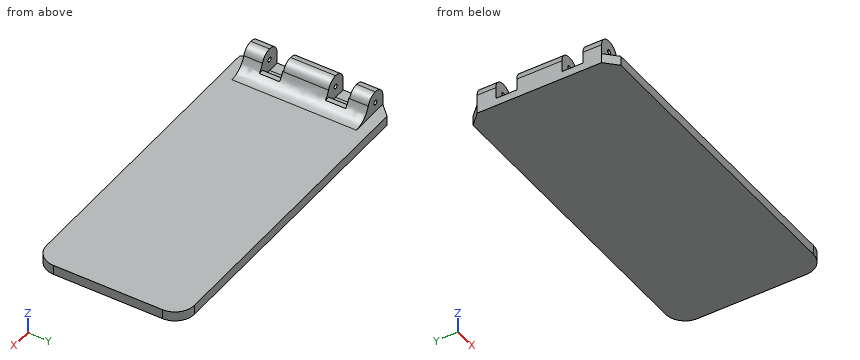
from build123d import *

# Parameters (mm, degrees)
BOSS_EXTRUDE1_DEPTH     = 38
FILLET1_R               = 5
CUT_EXTRUDE2_DEPTH      = 2.7
CUT_EXTRUDE2_DEPTH_BACK = 2.7
SKETCH4_R               = 3
CUT_EXTRUDE3_DEPTH      = 2.7
CUT_EXTRUDE3_DEPTH_BACK = 2.7
SKETCH5_R               = 3
SKETCH6_W               = 15.806991546
SKETCH6_H               = 7.262468959
CUT_EXTRUDE4_DEPTH      = 3
SKETCH7_W               = 28.198471628
SKETCH7_H               = 7.72700603
CUT_EXTRUDE5_DEPTH      = 3
CHAMFER1_SIZE           = 3
FILLET2_R               = 5
SKETCH8_W               = 6.878152115
SKETCH8_H               = 5.2
SKETCH8_W_2             = 6.400502662
CUT_EXTRUDE6_DEPTH      = 2


with BuildPart() as part:
    # Sketch1 → Boss-Extrude1 (new body)
    with BuildSketch(Plane(origin=(0, 0, 0), x_dir=(1, 0, 0), z_dir=(0, 1, 0))):
        with BuildLine():
            Line((85, 0), (3, 0))
            Line((3, 0), (3, -2))
            ThreePointArc((3, -2), (3.866025404, -2.127718677), (4.658312395, -2.5))
            Line((4.658312395, -2.5), (85, -2.5))
            Line((85, -2.5), (85, 0))
        make_face()
        with BuildLine():
            Line((3, -2), (3, 0))
            Line((3, 0), (0, 0))
            Line((0, 0), (0, -2.5))
            Line((0, -2.5), (1.341687605, -2.5))
            ThreePointArc((1.341687605, -2.5), (2.133974596, -2.127718677), (3, -2))
        make_face()
        with BuildLine():
            ThreePointArc((0, -5), (0.356617963, -3.581362835), (1.341687605, -2.5))
            Line((1.341687605, -2.5), (0, -2.5))
            Line((0, -2.5), (0, -5))
        make_face()
        with BuildLine():
            Line((3, -4.4), (3, -2.5))
            Line((3, -2.5), (0, -5))
            ThreePointArc((0, -5), (0.878679656, -7.121320344), (3, -8))
            Line((3, -8), (3, -5.6))
            ThreePointArc((3, -5.6), (2.4, -5), (3, -4.4))
        make_face()
        with BuildLine():
            Line((4.658312395, -2.5), (3, -2.5))
            Line((3, -2.5), (3, -4.4))
            ThreePointArc((3, -4.4), (3.424264069, -4.575735931), (3.6, -5))
            ThreePointArc((3.6, -5), (3.424264069, -5.424264069), (3, -5.6))
            Line((3, -5.6), (3, -8))
            ThreePointArc((3, -8), (5.121320344, -7.121320344), (6, -5))
            ThreePointArc((6, -5), (5.643382037, -3.581362835), (4.658312395, -2.5))
        make_face()
        with BuildLine():
            Line((0, -5), (3, -2.5))
            Line((3, -2.5), (1.341687605, -2.5))
            ThreePointArc((1.341687605, -2.5), (0.356617963, -3.581362835), (0, -5))
        make_face()
        with BuildLine():
            Line((3, -2.5), (3, -2))
            ThreePointArc((3, -2), (2.133974596, -2.127718677), (1.341687605, -2.5))
            Line((1.341687605, -2.5), (3, -2.5))
        make_face()
        with BuildLine():
            ThreePointArc((4.658312395, -2.5), (3.866025404, -2.127718677), (3, -2))
            Line((3, -2), (3, -2.5))
            Line((3, -2.5), (4.658312395, -2.5))
        make_face()
    extrude(amount=BOSS_EXTRUDE1_DEPTH)

    # Fillet1
    fillet1_edges = [part.edges().sort_by_distance(p)[0] for p in [
        (4.658312395, 19, 2.5),
    ]]
    fillet(fillet1_edges, radius=FILLET1_R)

    # Sketch4 → Cut-Extrude2 (cut, two sides: drawn at the far end of the back side and taken through both)
    with BuildSketch(Plane(origin=(0, 27.5, 0), x_dir=(1, 0, 0), z_dir=(0, 1, 0)).offset(-CUT_EXTRUDE2_DEPTH_BACK)):
        with Locations((3, -5)):
            Circle(SKETCH4_R)
        with BuildLine():
            ThreePointArc((0, -5), (0.878679656, -2.878679656), (3, -2))
            Line((3, -2), (0, -2))
            Line((0, -2), (0, -5))
        make_face()
    extrude(amount=CUT_EXTRUDE2_DEPTH + CUT_EXTRUDE2_DEPTH_BACK, mode=Mode.SUBTRACT)

    # Sketch5 → Cut-Extrude3 (cut, two sides: drawn at the far end of the back side and taken through both)
    with BuildSketch(Plane(origin=(0, 10.5, 0), x_dir=(1, 0, 0), z_dir=(0, 1, 0)).offset(-CUT_EXTRUDE3_DEPTH_BACK)):
        with Locations((3, -5)):
            Circle(SKETCH5_R)
        with BuildLine():
            ThreePointArc((0, -5), (0.878679656, -2.878679656), (3, -2))
            Line((3, -2), (0, -2))
            Line((0, -2), (0, -5))
        make_face()
    extrude(amount=CUT_EXTRUDE3_DEPTH + CUT_EXTRUDE3_DEPTH_BACK, mode=Mode.SUBTRACT)

    # Sketch6 → Cut-Extrude4 (cut)
    with BuildSketch(Plane(origin=(0, 38, 0), x_dir=(1, 0, 0), z_dir=(0, 1, 0))):
        with Locations((5.822770624, -6.13123448)):
            Rectangle(SKETCH6_W, SKETCH6_H)
    extrude(amount=-CUT_EXTRUDE4_DEPTH, mode=Mode.SUBTRACT)

    # Sketch7 → Cut-Extrude5 (cut)
    with BuildSketch(Plane.XZ):
        with Locations((11.372216332, 6.363503015)):
            Rectangle(SKETCH7_W, SKETCH7_H)
    extrude(amount=-CUT_EXTRUDE5_DEPTH, mode=Mode.SUBTRACT)

    # Chamfer1
    chamfer1_edges = [part.edges().sort_by_distance(p)[0] for p in [
        (0, 38, 1.25),
        (0, 0, 1.25),
    ]]
    chamfer(chamfer1_edges, length=CHAMFER1_SIZE)

    # Fillet2
    fillet2_edges = [part.edges().sort_by_distance(p)[0] for p in [
        (85, 38, 1.25),
        (85, 0, 1.25),
    ]]
    fillet(fillet2_edges, radius=FILLET2_R)

    # Sketch8 → Cut-Extrude6 (cut)
    with BuildSketch(Plane.XY.offset(5.9375)):
        with Locations((6.922338589, 10.4)):
            Rectangle(SKETCH8_W, SKETCH8_H)
        with Locations((6.683513862, 27.4)):
            Rectangle(SKETCH8_W_2, SKETCH8_H)
    extrude(amount=-CUT_EXTRUDE6_DEPTH, mode=Mode.SUBTRACT)


solid = part.part
Could you check a few things on this model? Use its own coordinates, in mm. Give positions to 0.01 mm unless a question says otherwise; leave off trailing zeros. Loops run counter-clockwise (first coordinate to the right, second up) from the corner with the lowest first, then second, coordinate; pieces in that order, holes last. Notation, with made-up numbers: M 26.5,24.5 L 85.5,24.5 A36 ccw 85.5,60.5 Z; hole C 72,-28 d8. An arc over 180 degrees is marked long. Answer as a JSON object with one key per item and string values.
Q1. Suppose I cut it at A-A, the plane z = 6.75. List the corners of the cut face in (x, y) for me, plus the area to 3 significant figures.
Values found:
{"outline": "M 0.56,3 L 5.44,3 L 5.44,7.8 L 0.56,7.8 Z; M 0.56,13.2 L 5.44,13.2 L 5.44,24.8 L 0.56,24.8 Z; M 0.56,30.2 L 5.44,30.2 L 5.44,35 L 0.56,35 Z", "area": "103 mm²"}
Q2. Suppose I cut it at B-B, the plane x = 50. List the corners of the cut face in (y, z) for me, plus the area to 3 significant figures.
Values found:
{"outline": "M 0,0 L 38,0 L 38,2.5 L 0,2.5 Z", "area": "95.0 mm²"}
Q3. If I drill on probe 1 along Y at (x, z) = (4, 7); probe 2 along Z at (x, y) = (24.5, 14); probe 3 along X at (y, z) = (7, 6), over which ranges is the centre line in solid material (lowest first)? Write a range as [from, to].
Values found:
{"probe 1": "y = [3, 7.8], [13.2, 24.8], [30.2, 35]", "probe 2": "z = [0, 2.5]", "probe 3": "x = [0.17, 5.83]"}
Q4. For P1, Ø6, axis at x = 41, y = 28.5, coming from the +Z side; P2, Ø1, axis at x = 6.5, z = 4.5, coming from the -Y side; P3, Ø1.8, axis at x = 5, z = 4.5, coming from the +Y side, each with a flat end and sliding along its axis, tell me the tip position at first contact or that it passes through.
Values found:
{"P1": "stops at z = 2.5", "P2": "stops at y = 3", "P3": "stops at y = 35"}
